from build123d import *

# Parameters (mm, degrees)
F0_R     = 38.1
F0_R_2   = 2.37453
F0_R_3   = 25.404017
F1_DEPTH = 6.35
F2_R     = 25.338119
F3_DEPTH = 12.7
F4_R     = 19.05
F5_DEPTH = 12.7
F6_R     = 12.7
F7_DEPTH = 25.4


with BuildPart() as f1:
    # F0 (on Top) → F1 (new body)
    with BuildSketch(Plane.XY):
        Circle(F0_R)
        with Locations((-9.525, -31.75)):
            Circle(F0_R_2, mode=Mode.SUBTRACT)
        with Locations((9.525, -31.75)):
            Circle(F0_R_2, mode=Mode.SUBTRACT)
        with Locations((-9.525, 31.75)):
            Circle(F0_R_2, mode=Mode.SUBTRACT)
        Circle(F0_R_3, mode=Mode.SUBTRACT)
        with Locations((9.525, 31.75)):
            Circle(F0_R_2, mode=Mode.SUBTRACT)
        Circle(F0_R_3)
    extrude(amount=F1_DEPTH)

    # F2 (on face) → F3 (join)
    with BuildSketch(Plane.XY.offset(6.35)):
        Circle(F2_R)
    extrude(amount=F3_DEPTH)

    # F4 (on face) → F5 (cut)
    with BuildSketch(Plane(origin=(0, 0, 0), x_dir=(1, 0, 0), z_dir=(0, 0, -1))):
        Circle(F4_R)
    extrude(amount=-F5_DEPTH, mode=Mode.SUBTRACT)

    # F6 (on face) → F7 (cut)
    with BuildSketch(Plane.XY.offset(19.05)):
        Circle(F6_R)
    extrude(amount=-F7_DEPTH, mode=Mode.SUBTRACT)


solid = f1.part
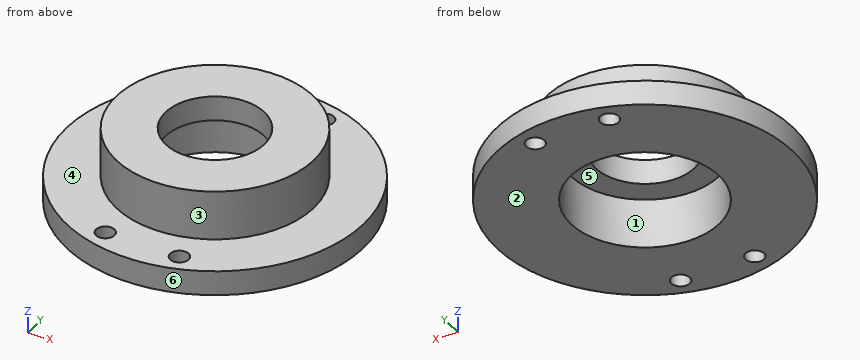
Design review of the part built by this model. Coordinates are the model's own, in mm. Face numbers are marked on the shaded views. A direction names the side the tool comes from. Round coordinates to 2 decimals unless told otherwise and drop trailing zeros. Loops run counter-clockwise (first coordinate to the right, second up) from the corner with the lowest first, then second, coordinate; pieces in that order, holes last. Notation, with made-up numbers: (37, 16) - (93, 16) arc R30 ccw to (93, 46) - close; hole circle Ø4 at (39, 87.5). An arc over 180 degrees is marked (long way). One line per item, written item: value. Start each with the question number.
1) To check wall thickness, follow L1, parallel to Y at x = 10.5, z = 4; L2, parallel to Y at x = 0, z = 5.75; L3, parallel to Y at x = 0, z = 6.75. State the ranges of each line that lie inside material, in increasing order. Write a range as from..to.
2) For the marked faces 1, 2 and 3, list the 3-axis set-ups (+Z, -Z, +X, -X, +Y, -Y) from which the entire face can be reached by the end or side of a thin tool; tool diameter is ignored.
3) Insertion check: pin 1 Ø6 at (x, y) = (9.525, -31.75) entering from -Z; pin 2 Ø5.5 at (x, y) = (-9.525, -31.75) entering from +Z; pin 3 Ø4 at (x, z) = (-12, 10) entering from +Y; pin 4 Ø4 at (y, z) = (-7.5, 2.5) entering from -X. Each pin has a flat end and moves straight along its axis. Give the tip position at first contact, or say it passes through.
4) Consider section C-C on z = 3.75. Give the boundary of the cut face in (x, y) (3 decimals), then the cut area to 3 significant figures.
5) Draft analysis for pull direction X (two halves, no side actions). For the marked faces 4, 5 and 6, state which applies: +X half, -X half, draft (parallel to the pull), parting line (faces both ways), or undercut.
6) Consider section A-A on x = 0. Give the boundary of the cut face in (y, z).
7) Consider section D-D on y = 33. Give the boundary of the cut face in (x, z).
Reported:
1. L1: y = -36.62..-33.92, -29.58..-15.9, 15.9..29.58, 33.92..36.62
1. L2: y = -38.1..-19.05, 19.05..38.1
1. L3: y = -25.34..-19.05, 19.05..25.34
2. face 1: -Z
2. face 2: -Z, +X, -X, +Y, -Y
2. face 3: +Z
3. pin 1: stops at z = 0
3. pin 2: stops at z = 6.35
3. pin 3: stops at y = 23.28
3. pin 4: stops at x = -37.7
4. outline: circle Ø76.2 at (0, 0); hole circle Ø38.1 at (0, 0); hole circle Ø4.749 at (-9.525, -31.75); hole circle Ø4.749 at (-9.525, 31.75); hole circle Ø4.749 at (9.525, -31.75); hole circle Ø4.749 at (9.525, 31.75)
4. area: 3,350 mm^2
5. face 4: draft
5. face 5: undercut
5. face 6: parting line
6. outline: (-38.1, 0) - (-19.05, 0) - (-19.05, 12.7) - (-12.7, 12.7) - (-12.7, 19.05) - (-25.34, 19.05) - (-25.34, 6.35) - (-38.1, 6.35) - close; (12.7, 12.7) - (19.05, 12.7) - (19.05, 0) - (38.1, 0) - (38.1, 6.35) - (25.34, 6.35) - (25.34, 19.05) - (12.7, 19.05) - close
7. outline: (-19.04, 0) - (-11.54, 0) - (-11.54, 6.35) - (-19.04, 6.35) - close; (-7.51, 0) - (7.51, 0) - (7.51, 6.35) - (-7.51, 6.35) - close; (11.54, 0) - (19.04, 0) - (19.04, 6.35) - (11.54, 6.35) - close
